Verification items for this drawing (mm, ordinates from the low corner). Give positions to 0.01 mm unless a question says otherwise; leave off trailing zeros. Loops run counter-clockwise (first coordinate to the right, second up) from the corner with the lowest first, then second, coordinate; pieces in that order, holes last. Notation, with made-up numbers: (15, 19.25) -> (55, 19.25) arc R20 ccw to (55, 56.25) -> close; hole circle Ø8 at (87.25, 27). An arc over 180 degrees is marked (long way). Write item = value, one per line.
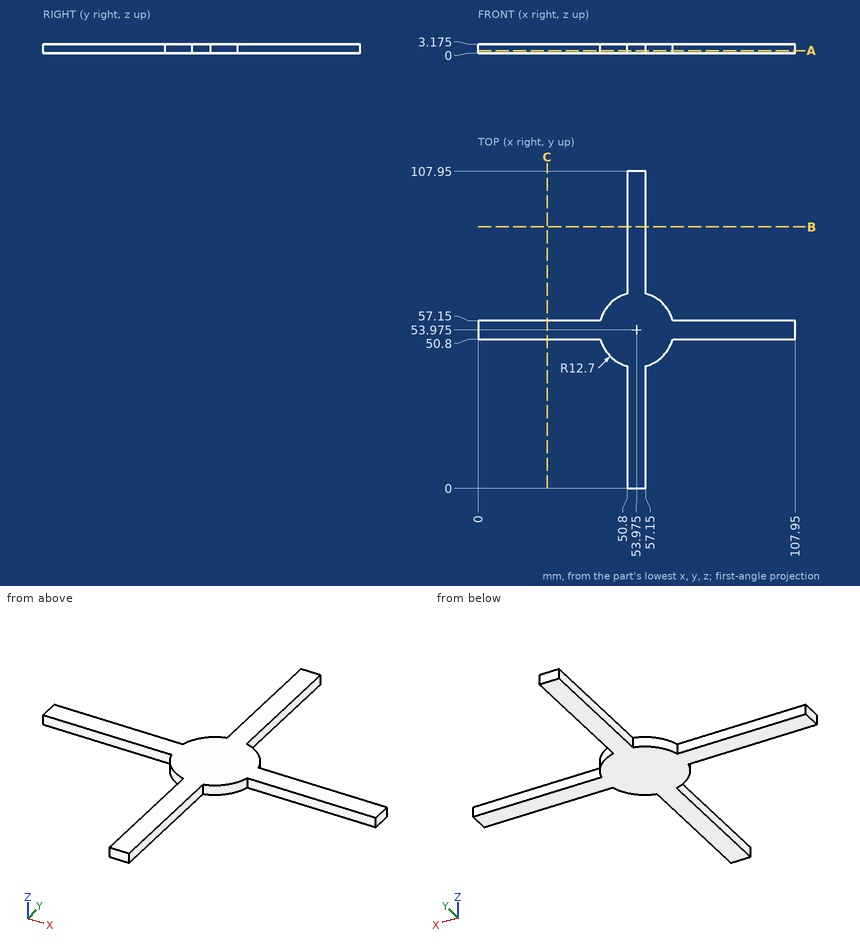
Item 1: Gauge pin test, flat ends, axial feed: pin 1 (1 mm diameter, centred on x = 85, z = 2, fed in from +Y); pin 2 (1.6 mm diameter, centred on x = 15.5, z = 2, fed in from -Y); pin 3 (1.6 mm diameter, centred on y = 17.5, z = 1.5, fed in from -X). Record the tip position at first contact, or that the pin passes through.
Answer:
pin_1 = 57.15
pin_2 = 50.8
pin_3 = 50.8
Item 2: Thickness scan on L1, parallel to X at y = 17.5, z = 2.9. Record the ranges inside material, lowest first. Write a range as [from, to].
Answer:
L1 = [50.8, 57.15]
Item 3: Section check A-A, the plane z = 0.9. Record the cut outline in (x, y) (3 decimals).
Answer:
outline = (0, 50.8) -> (41.678, 50.8) arc R12.7 ccw to (50.8, 41.678) -> (50.8, 0) -> (57.15, 0) -> (57.15, 41.678) arc R12.7 ccw to (66.272, 50.8) -> (107.95, 50.8) -> (107.95, 57.15) -> (66.272, 57.15) arc R12.7 ccw to (57.15, 66.272) -> (57.15, 107.95) -> (50.8, 107.95) -> (50.8, 66.272) arc R12.7 ccw to (41.678, 57.15) -> (0, 57.15) -> close
Item 4: Section check B-B, the plane y = 89. Record the cut outline in (x, z) (3 decimals).
Answer:
outline = (50.8, 0) -> (57.15, 0) -> (57.15, 3.175) -> (50.8, 3.175) -> close
